Autodesk Inventor part; units mm, degrees
ref_plane "YZ Plane" through (0, 0, 0) normal (1, 0, 0) x (0, 1, 0)
ref_plane "XZ Plane" through (0, 0, 0) normal (0, 1, 0) x (-1, 0, 0)
ref_plane "XY Plane" through (0, 0, 0) normal (0, 0, 1) x (1, 0, 0)
sketch "Sketch1" plane through (0, 0, 0) normal (0, 1, 0) x (-1, 0, 0)
  circle A0 centre (0, 0) radius 16
  dimension "d0" = 32
extrude "Extrusion1" add sketch "Sketch1" along normal blind 19.5
sketch "Sketch2" plane through (0, 19.5, 0) normal (0, 1, 0) x (1, 0, 0)
  circle A0 centre (0, 0) radius 16
  circle A1 centre (0, 0) radius 3.1
  dimension "d3" = 6.2
extrude "Extrusion2" add sketch "Sketch2" along normal blind 1.9 contours A1
sketch "Sketch3" plane through (0, 21.4, 0) normal (0, 1, 0) x (1, 0, 0)
  circle A0 centre (0, 0) radius 3.1
  circle A1 centre (0, 0) radius 1
  dimension "d6" = 2
extrude "Extrusion3" add sketch "Sketch3" along normal blind 22 contours A1
sketch "Sketch4" plane through (0, 19.5, 0) normal (0, 1, 0) x (1, 0, 0)
  circle A0 centre (0, 0) radius 3.1
  circle A1 centre (0, 0) radius 16
  circle A2 centre (0, -11) radius 1.3
  circle A3 centre (0, 11) radius 1.3
  line L0 (-16, 0) -> (16, 0)
  dimension "d9" = 2.6
  dimension "d10" = 22
extrude "Extrusion4" cut sketch "Sketch4" against normal blind 4 contours A2 | A3
fillet "Fillet1" radius 0.9 1 edges at (16, 19.5, 0)
properties part number "rf500tb"
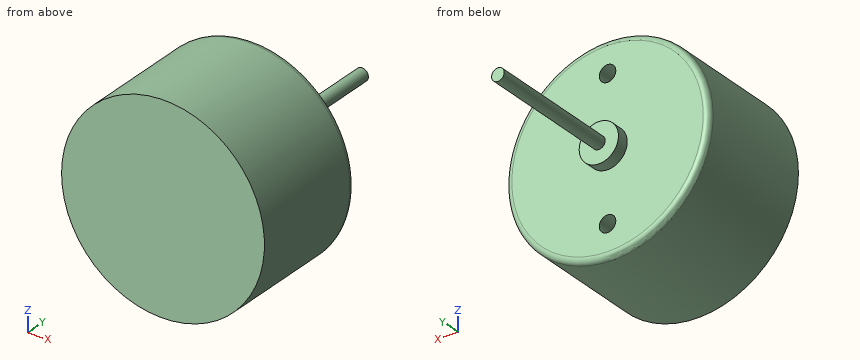
Part model, mm, in its own coordinate system. Round coordinates to 2 decimals unless told otherwise and drop trailing zeros. Write each loop counter-clockwise with the first axis right and the second up, starting at its lowest first coordinate (ties: lowest second). Pieces come first, ordered by that corner, then holes. Notation, with made-up numbers: M 64.25,-18.5 L 122.25,-18.5 A23 ccw 122.25,4.5 Z; hole C 43,31.5 d11. An arc over 180 degrees is marked long. One line per question, with ' | ' between items.
(1) Saw through at A-A on x = 0. Write the cut outline in (y, z).
Answer key:
outline: M 0,-16 L 18.6,-16 A0.9 ccw 19.5,-15.1 L 19.5,-12.3 L 15.5,-12.3 L 15.5,-9.7 L 19.5,-9.7 L 19.5,-3.1 L 21.4,-3.1 L 21.4,-1 L 43.4,-1 L 43.4,1 L 21.4,1 L 21.4,3.1 L 19.5,3.1 L 19.5,9.7 L 15.5,9.7 L 15.5,12.3 L 19.5,12.3 L 19.5,15.1 A0.9 ccw 18.6,16 L 0,16 Z
(2) Saw through at C-C on y = 11. Write the cut outline in (x, z).
Answer key:
outline: C 0,0 d32
(3) Pin check, flat tips, straight feed: pin 1 (2 mm diameter, centred on x = -12.5, z = 6, fed in from -Y); pin 2 (1.6 mm diameter, centred on x = 0, z = 11, fed in from +Y); pin 3 (10 mm diameter, centred on y = 14.5, z = -6.5, fed in from +X); pin 4 (1 mm diameter, centred on x = -11.5, z = -5.5, fed in from +Y). Stop position of each tip, or through.
Answer key:
pin 1: stops at y = 0 | pin 2: stops at y = 15.5 | pin 3: stops at x = 15.93 | pin 4: stops at y = 19.5
(4) Saw through at B-B on z = 0. Write the cut outline in (x, y).
Answer key:
outline: M -16,0 L 16,0 L 16,18.6 A0.9 ccw 15.1,19.5 L 3.1,19.5 L 3.1,21.4 L 1,21.4 L 1,43.4 L -1,43.4 L -1,21.4 L -3.1,21.4 L -3.1,19.5 L -15.1,19.5 A0.9 ccw -16,18.6 Z
(5) Saw through at D-D on y = 35. Write the cut outline in (x, z).
Answer key:
outline: C 0,0 d2
(6) Probe line 1 along Z through (x, y) = (0, 16.5); line 2 along Y through (x, z) = (2, 13); line 3 along X through (y, z) = (18.55, 11). List the from-to ranges inside material, lowest first.
Answer key:
line 1: z = -16 to -12.3, -9.7 to 9.7, 12.3 to 16 | line 2: y = 0 to 19.5 | line 3: x = -11.62 to -1.3, 1.3 to 11.62
